Read the model definition and answer for the solid it produces. Units are mm, in the model's axes. Face numbers are marked on the shaded views. A direction names the side the tool comes from. Give positions to 0.01 mm unless a question says otherwise; leave off trailing zeros. Order: outer loops, then holes, each group sorted by start corner. A loop starts at its lowest first (then second) coordinate and runs counter-clockwise, first axis right, second up. Notation, with made-up numbers: (76, 80.25) - (93, 80.25) arc R25 ccw to (93, 114.25) - close; hole circle Ø10 at (82.5, 77.25). An arc over 180 degrees is marked (long way). Write item = value, one per line.
Autodesk Inventor part; units mm, degrees
ref_plane "YZ Plane" through (0, 0, 0) normal (1, 0, 0) x (0, 1, 0)
ref_plane "XZ Plane" through (0, 0, 0) normal (0, 1, 0) x (-1, 0, 0)
ref_plane "XY Plane" through (0, 0, 0) normal (0, 0, 1) x (1, 0, 0)
sketch "Sketch1" plane through (0, 0, 0) normal (0, 0, 1) x (1, 0, 0)
  line L0 (-37.5, -25) -> (37.5, -25)
  line L1 (37.5, -25) -> (37.5, 25)
  line L2 (37.5, 25) -> (-37.5, 25)
  line L3 (-37.5, 25) -> (-37.5, -25)
  line L4 (-37.5, -25) -> (37.5, 25) construction
  line L5 (37.5, -25) -> (-37.5, 25) construction
  line L6 (-15.1, 25) -> (15.1, 25)
  line L7 (15.1, 25) -> (15.1, 20)
  line L8 (15.1, 20) -> (-15.1, 20)
  line L9 (-15.1, 20) -> (-15.1, 25)
  line L10 (-15.1, 25) -> (15.1, 20) construction
  line L11 (15.1, 25) -> (-15.1, 20) construction
  line L12 (-4.9474, -25) -> (-37.5, -25)
  line L13 (-37.5, -25) -> (-37.5, -21.6221)
  line L14 (74.3708, -25) -> (124.7526, -25)
  line L15 (0, 0) -> (0, -25) construction
  line L16 (24.4526, -25) -> (37.5, -25)
  line L17 (37.5, -25) -> (37.5, -19.8)
  line L18 (-10, 0) -> (10, 0) construction
  line L19 (-10, -6) -> (10, -6)
  line L20 (10, 6) -> (-10, 6)
  arc A0 (-10, 6) -> (-10, -6) centre (-10, 0) ccw
  arc A1 (10, -6) -> (10, 6) centre (10, 0) ccw
  line L21 (-2.5, 6) -> (2.5, 6)
  line L22 (2.5, 6) -> (2.5, 20)
  line L23 (2.5, 20) -> (-2.5, 20)
  line L24 (-2.5, 20) -> (-2.5, 6)
  line L25 (-2.5, 6) -> (2.5, 20) construction
  line L26 (2.5, 6) -> (-2.5, 20) construction
  line L27 (-37.5, -25) -> (-20.5763, -25)
  line L28 (-37.5, -20) -> (-37.5, -25)
  line L29 (20.5763, -25) -> (37.5, -25)
  line L30 (37.5, -25) -> (37.5, -20)
  line L31 (-15, -25) -> (15, -25)
  line L32 (15, -25) -> (15, -20)
  line L33 (15, -20) -> (-15, -20) construction
  line L34 (-15, -20) -> (-15, -25)
  line L35 (-15, -25) -> (15, -20) construction
  line L36 (15, -25) -> (-15, -20) construction
  line L37 (-15, -20) -> (-37.5, -20)
  line L38 (15, -20) -> (37.5, -20)
  point P0 (0, 22.5)
  point P1 (15.1, 25)
  point P2 (-15.1, 25)
  point P3 (0, 13)
  point P4 (2.5, 20)
  point P5 (0, -22.5)
  dimension "d1" = 50
  dimension "d10" = 5
  dimension "d11" = 30.2
  dimension "d25" = 12
  dimension "d26" = 20
  dimension "d27" = 5
  dimension "d35" = 5
  dimension "d36" = 30
  dimension "d37" = 75
extrude "Extrusion1" add sketch "Sketch1" along normal blind 5 contours L34 L37 L3 L2 L9 L8 L24 L20 A0 L19 A1 L22 L7 L1 L38 L32 L0
properties part number "upper-back-plate-support"
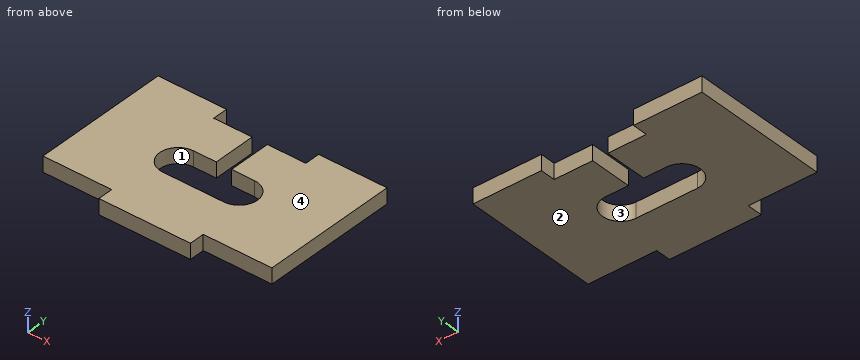
1. Flat-ended cylindrical pins translate along their axes: pin 1 (1.5 mm diameter, centred on x = -9.5, z = 1.5, fed in from +Y); pin 2 (2.5 mm diameter, centred on x = -27.5, z = 2.5, fed in from -Y); pin 3 (1 mm diameter, centred on x = 28.5, y = 4.5, fed in from -Z); pin 4 (2.5 mm diameter, centred on y = -22.5, z = 3.5, fed in from -X). Find the tip coordinate at first contact, or state that the pin passes through.
Recorded:
pin_1 = 20
pin_2 = -20
pin_3 = 0
pin_4 = -15
2. For the marked faces 1 and 2, determine the directions among +Z, -Z, +X, -X, +Y, -Y from which every point of the face is accessible in a straight line to the end or side of a thin tool.
Recorded:
face_1 = +Z, -Z
face_2 = -Z, +X, -X, +Y, -Y
3. Section A-A (x = 5) is taken. Determine the outline of the cut face in (y, z).
Recorded:
outline = (-25, 0) - (-6, 0) - (-6, 5) - (-25, 5) - close; (6, 0) - (20, 0) - (20, 5) - (6, 5) - close
4. Determine the mould class of the marked faces 3 and 4 for opening direction Y: +Y half, -Y half, draft (parallel to the pull), parting line (faces both ways), or undercut.
Recorded:
face_3 = undercut
face_4 = draft
5. Straight lines are drawn through the part: L1, parallel to X at y = 17.5, z = 4.8; L2, parallel to X at y = 20.5, z = 1.7; L3, parallel to Y at x = 4, z = 4.4. For each, find the intervals that lie inside material, in ascending order. Write a range as [from, to].
Recorded:
L1 = [-37.5, -2.5], [2.5, 37.5]
L2 = [-37.5, -15.1], [15.1, 37.5]
L3 = [-25, -6], [6, 20]
6. Section C-C (z = 2.6) is taken. Determine the outline of the cut face in (x, y).
Recorded:
outline = (-37.5, -20) - (-15, -20) - (-15, -25) - (15, -25) - (15, -20) - (37.5, -20) - (37.5, 25) - (15.1, 25) - (15.1, 20) - (2.5, 20) - (2.5, 6) - (10, 6) arc R6 cw to (10, -6) - (-10, -6) arc R6 cw to (-10, 6) - (-2.5, 6) - (-2.5, 20) - (-15.1, 20) - (-15.1, 25) - (-37.5, 25) - close
7. Section D-D (x = 20) is taken. Determine the outline of the cut face in (y, z), and give its area (3 significant figures).
Recorded:
outline = (-20, 0) - (25, 0) - (25, 5) - (-20, 5) - close
area = 225 mm^2
8. Section B-B (y = 0) is taken. Determine the outline of the cut face in (x, z), and give its area (3 significant figures).
Recorded:
outline = (-37.5, 0) - (-16, 0) - (-16, 5) - (-37.5, 5) - close; (16, 0) - (37.5, 0) - (37.5, 5) - (16, 5) - close
area = 215 mm^2
